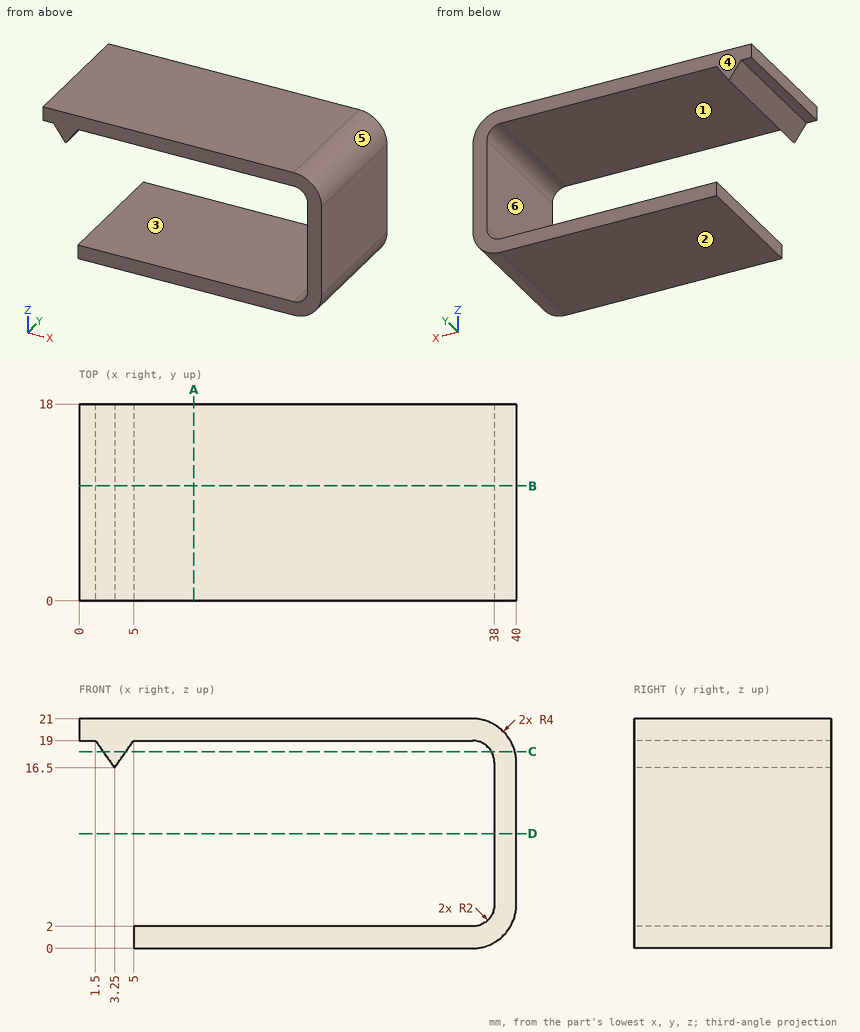
The figure shows three views and two pictorial views of one solid part (mm, origin at its lowest corner). Answer the questions. A direction names the side the tool comes from. Give positions to 0.01 mm unless a question says otherwise; leave off trailing zeros. Write each loop counter-clockwise with the first axis right and the second up, starting at its lowest first coordinate (ties: lowest second). Pieces come first, ordered by that corner, then holes. Notation, with made-up numbers: (82.25, -5) -> (101.25, -5) arc R7 cw to (101.25, 7) -> close; hole circle Ø4 at (-40, 39). An arc over 180 degrees is marked (long way). Use one line per item in the form item = value.
1) Section C-C on z = 18 is taken. Write down the section's boundary in (x, y), plus the area to 3 significant figures.
Result:
outline = (2.2, 0) -> (4.3, 0) -> (4.3, 18) -> (2.2, 18) -> close; (37.73, 0) -> (39.87, 0) -> (39.87, 18) -> (37.73, 18) -> close
area = 76.3 mm²
2) Straight lines are drawn through the part: probe 1 along Z at (x, y) = (26, 12.75); probe 2 along X at (y, z) = (12, 4); probe 3 along Z at (x, y) = (36.5, 14.5). For each, find the intervals that lie inside material, in ascending order.
Result:
probe_1 = 0 to 2, 19 to 21
probe_2 = 38 to 40
probe_3 = 0.03 to 2.06, 18.94 to 20.97
3) For a pull along Z with two mould halves and no side action, classify the marked faces 4, 5 and 6 as +Z half, -Z half, draft (parallel to the pull), parting line (faces both ways), or undercut.
Result:
face_4 = draft
face_5 = +Z half
face_6 = undercut
4) Each of these flat-tipped pins is pushed along its axis until it touches: P1, Ø1.6, axis at x = 0.5, y = 5.5, coming from the -Z side; P2, Ø1.6, axis at y = 5.5, z = 0.5, coming from the -X side. Where does it stop, or does it pass through?
Result:
P1 = 19
P2 = 5
5) A tool of negligible diameter and unlimited length cuts with its end or side. For the marked faces 1, 2 and 3, from which of +Z, -Z, +X, -X, +Y, -Y can it reach the whole face along a straight path? Write none if from no direction.
Result:
face_1 = +Y, -Y
face_2 = -Z, +X, -X, +Y, -Y
face_3 = -X, +Y, -Y
6) Section A-A on x = 10.5 is taken. Write down the section's boundary in (y, z), plus the area to 3 significant figures.
Result:
outline = (0, 0) -> (18, 0) -> (18, 2) -> (0, 2) -> close; (0, 19) -> (18, 19) -> (18, 21) -> (0, 21) -> close
area = 72.0 mm²
7) Section D-D on z = 10.5 is taken. Write down the section's boundary in (x, y), plus the area to 3 significant figures.
Result:
outline = (38, 0) -> (40, 0) -> (40, 18) -> (38, 18) -> close
area = 36.0 mm²
8) Section B-B on y = 10.5 is taken. Write down the section's boundary in (x, z).
Result:
outline = (0, 19) -> (1.5, 19) -> (3.25, 16.5) -> (5, 19) -> (36, 19) arc R2 cw to (38, 17) -> (38, 4) arc R2 cw to (36, 2) -> (5, 2) -> (5, 0) -> (36, 0) arc R4 ccw to (40, 4) -> (40, 17) arc R4 ccw to (36, 21) -> (0, 21) -> close
